Design review of the part built by this model. Coordinates are the model's own, in mm. Face numbers are marked on the shaded views. A direction names the side the tool comes from. Round coordinates to 2 decimals unless told otherwise and drop trailing zeros. Loops run counter-clockwise (first coordinate to the right, second up) from the corner with the lowest first, then second, coordinate; pieces in that order, holes last. Notation, with made-up numbers: (10.25, 66) -> (68.25, 66) arc R12 cw to (68.25, 72) -> close; hole circle Ø3 at (72, -33.75). An arc over 180 degrees is marked (long way). Answer as CSV lines item,"result". Start each with the question number.
(1) Take a section at B-B, the plane x = 0. Write out the cut boundary in (y, z), and give its area (3 significant figures).
(2) Take a section at C-C, the plane x = 11. Write out the cut boundary in (y, z), and give its area (3 significant figures).
(3) For P1, Ø6, axis at x = 8, z = 247, coming from the -Y side; P2, Ø1.8, axis at x = 0.5, y = 71.5, coming from the +Z side; P3, Ø1.5, axis at y = 74.5, z = 244, coming from the +X side, all flat-tipped, find the tip position at first contact; note any pin that passes through.
(4) Take a section at A-A, the plane y = 83. Write out the cut boundary in (x, z).
(5) To check wall thickness, follow line 1 (Y direction, x = 0, z = 251.2); line 2 (Y direction, x = 0.5, z = 246.25); line 3 (Z direction, x = 1.5, y = 95). State the ranges of each line that lie inside material, in increasing order. Write a range as from..to.
(6) Take a section at D-D, the plane y = 94. Write out the cut boundary in (x, z).
(7) Machinability: for the marked faces 4 and 5, which of the approach directions +Z, -Z, +X, -X, +Y, -Y give a long, thin tool a straight path to every point of the face, cutting with its end or side? Answer none if there is none.
(8) Draft analysis for pull direction Y (two halves, no side actions). For the marked faces 1, 2 and 3, state which applies: +Y half, -Y half, draft (parallel to the pull), parting line (faces both ways), or undercut.
from build123d import *

# Parameters (mm, degrees)
CYLINDER672_R     = 2.65
CYLINDER672_DEPTH = 30
CYLINDER664_R     = 3
CYLINDER664_DEPTH = 3
CYLINDER661_R     = 3
CYLINDER661_DEPTH = 3
CYLINDER668_R     = 3
CYLINDER668_DEPTH = 3
CYLINDER666_R     = 3
CYLINDER666_DEPTH = 3
CYLINDER673_R     = 1.5
CYLINDER673_DEPTH = 30
CYLINDER658_R     = 1.5
CYLINDER658_DEPTH = 30
CYLINDER671_R     = 1.5
CYLINDER671_DEPTH = 30
CYLINDER667_R     = 1.5
CYLINDER667_DEPTH = 30
CYLINDER665_R     = 15.1
CYLINDER665_DEPTH = 10


with BuildPart() as obj1:
    # Cylinder672 → Cylinder672 (new body)
    with BuildSketch(Plane(origin=(0, 83, 232), x_dir=(1, 0, 0), z_dir=(0, 0, 1))):
        Circle(CYLINDER672_R)
    extrude(amount=CYLINDER672_DEPTH)


with BuildPart() as obj2:
    # Cylinder664 → Cylinder664 (new body)
    with BuildSketch(Plane(origin=(11, 83, 232), x_dir=(1, 0, 0), z_dir=(0, 0, 1))):
        Circle(CYLINDER664_R)
    extrude(amount=CYLINDER664_DEPTH)


with BuildPart() as obj3:
    # Cylinder661 → Cylinder661 (new body)
    with BuildSketch(Plane(origin=(0, 72, 232), x_dir=(1, 0, 0), z_dir=(0, 0, 1))):
        Circle(CYLINDER661_R)
    extrude(amount=CYLINDER661_DEPTH)


with BuildPart() as obj4:
    # Cylinder668 → Cylinder668 (new body)
    with BuildSketch(Plane(origin=(0, 94, 232), x_dir=(1, 0, 0), z_dir=(0, 0, 1))):
        Circle(CYLINDER668_R)
    extrude(amount=CYLINDER668_DEPTH)


with BuildPart() as compound362:
    # Cylinder666 → Cylinder666 (new body)
    with BuildSketch(Plane(origin=(-11, 83, 232), x_dir=(1, 0, 0), z_dir=(0, 0, 1))):
        Circle(CYLINDER666_R)
    extrude(amount=CYLINDER666_DEPTH)

    # Compound362: union obj2, obj3, obj4
    add(obj2.part)
    add(obj3.part)
    add(obj4.part)


with BuildPart() as compound362_1:
    # Compound362 placement: moved
    add(compound362.part.moved(Location((0, 0, 17))))


with BuildPart() as obj5:
    # Cylinder673 → Cylinder673 (new body)
    with BuildSketch(Plane(origin=(11, 83, 232), x_dir=(1, 0, 0), z_dir=(0, 0, 1))):
        Circle(CYLINDER673_R)
    extrude(amount=CYLINDER673_DEPTH)


with BuildPart() as obj6:
    # Cylinder658 → Cylinder658 (new body)
    with BuildSketch(Plane(origin=(0, 72, 232), x_dir=(1, 0, 0), z_dir=(0, 0, 1))):
        Circle(CYLINDER658_R)
    extrude(amount=CYLINDER658_DEPTH)


with BuildPart() as obj7:
    # Cylinder671 → Cylinder671 (new body)
    with BuildSketch(Plane(origin=(0, 94, 232), x_dir=(1, 0, 0), z_dir=(0, 0, 1))):
        Circle(CYLINDER671_R)
    extrude(amount=CYLINDER671_DEPTH)


with BuildPart() as compound361:
    # Cylinder667 → Cylinder667 (new body)
    with BuildSketch(Plane(origin=(-11, 83, 232), x_dir=(1, 0, 0), z_dir=(0, 0, 1))):
        Circle(CYLINDER667_R)
    extrude(amount=CYLINDER667_DEPTH)

    # Compound361: union obj5, obj6, obj7
    add(obj5.part)
    add(obj6.part)
    add(obj7.part)


with BuildPart() as cut267:
    # Cylinder665 → Cylinder665 (new body)
    with BuildSketch(Plane(origin=(0, 83, 242), x_dir=(1, 0, 0), z_dir=(0, 0, 1))):
        Circle(CYLINDER665_R)
    extrude(amount=CYLINDER665_DEPTH)

    # Cut269: cut Compound361
    add(compound361.part, mode=Mode.SUBTRACT)

    # Cut270: cut Compound362
    add(compound362_1.part, mode=Mode.SUBTRACT)

    # Cut267: cut obj1
    add(obj1.part, mode=Mode.SUBTRACT)


solid = cut267.part
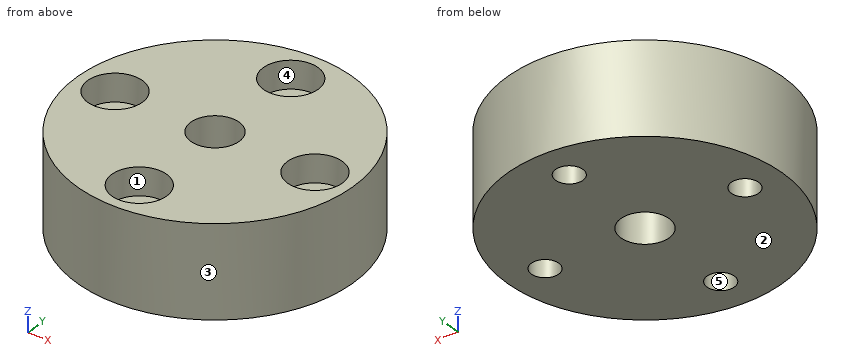
The answers:
1,outline,"(67.9, 242) -> (70.5, 242) -> (70.5, 249) -> (69, 249) -> (69, 252) -> (67.9, 252) -> close; (73.5, 242) -> (80.35, 242) -> (80.35, 252) -> (75, 252) -> (75, 249) -> (73.5, 249) -> close; (85.65, 242) -> (92.5, 242) -> (92.5, 249) -> (91, 249) -> (91, 252) -> (85.65, 252) -> close; (95.5, 242) -> (98.1, 242) -> (98.1, 252) -> (97, 252) -> (97, 249) -> (95.5, 249) -> close"
1,area,"171 mm²"
2,outline,"(72.66, 242) -> (81.5, 242) -> (81.5, 249) -> (80, 249) -> (80, 252) -> (72.66, 252) -> close; (84.5, 242) -> (93.34, 242) -> (93.34, 252) -> (86, 252) -> (86, 249) -> (84.5, 249) -> close"
2,area,"168 mm²"
3,P1,"y = 68.75"
3,P2,"z = 249"
3,P3,"x = 12.96"
4,outline,"(-15.1, 242) -> (-12.5, 242) -> (-12.5, 249) -> (-14, 249) -> (-14, 252) -> (-15.1, 252) -> close; (-9.5, 242) -> (-2.65, 242) -> (-2.65, 252) -> (-8, 252) -> (-8, 249) -> (-9.5, 249) -> close; (2.65, 242) -> (9.5, 242) -> (9.5, 249) -> (8, 249) -> (8, 252) -> (2.65, 252) -> close; (12.5, 242) -> (15.1, 242) -> (15.1, 252) -> (14, 252) -> (14, 249) -> (12.5, 249) -> close"
5,line 1,"67.9..69, 75..80.35, 85.65..91, 97..98.1"
5,line 2,"67.91..70.59, 73.41..80.4, 85.6..92.59, 95.41..98.09"
5,line 3,"242..249"
6,outline,"(-10.34, 242) -> (-1.5, 242) -> (-1.5, 249) -> (-3, 249) -> (-3, 252) -> (-10.34, 252) -> close; (1.5, 242) -> (10.34, 242) -> (10.34, 252) -> (3, 252) -> (3, 249) -> (1.5, 249) -> close"
7,face 4,"+Z"
7,face 5,"+Z, -Z"
8,face 1,"undercut"
8,face 2,"draft"
8,face 3,"parting line"
